from build123d import *

# Parameters (mm, degrees)
SKETCH1_W                        = 55.245
SKETCH1_H                        = 36.15436
BOSS_EXTRUDE1_DEPTH              = 3.175
SKETCH7_W                        = 3.302
SKETCH7_H                        = 19.177
CUT_EXTRUDE1_DEPTH               = 3.175
FILLET1_R                        = 6.35
F_10_0_1935_DIAMETER_HOLE2_D     = 4.9149
F_10_0_1935_DIAMETER_HOLE2_DEPTH = 9.699415072
F_10_0_1935_DIAMETER_HOLE2_TIP   = 1.476584928


with BuildPart() as part:
    # Sketch1 → Boss-Extrude1 (new body)
    with BuildSketch(Plane(origin=(0, 0, 0), x_dir=(0, 0, -1), z_dir=(1, 0, 0))):
        with Locations((27.6225, 18.07718)):
            Rectangle(SKETCH1_W, SKETCH1_H)
    extrude(amount=BOSS_EXTRUDE1_DEPTH)

    # Sketch7 → Cut-Extrude1 (cut)
    with BuildSketch(Plane.ZY):
        with Locations((-43.469153092, 20.34286)):
            Rectangle(SKETCH7_W, SKETCH7_H)
        with Locations((-17.942153092, 20.34286)):
            Rectangle(SKETCH7_W, SKETCH7_H)
    extrude(amount=-CUT_EXTRUDE1_DEPTH, mode=Mode.SUBTRACT)

    # Fillet1
    fillet1_edges = [part.edges().sort_by_distance(p)[0] for p in [
        (1.5875, 0, 0),
        (1.5875, 36.15436, 0),
        (1.5875, 36.15436, -55.245),
        (1.5875, 0, -55.245),
    ]]
    fillet(fillet1_edges, radius=FILLET1_R)

    # #10 (0.1935) Diameter Hole2
    with Locations(Plane.ZY):
        with Locations((-30.642153092, 9.525), (-30.642153092, 26.67), (-6.829653092, 9.525)):
            Hole(F_10_0_1935_DIAMETER_HOLE2_D / 2, depth=F_10_0_1935_DIAMETER_HOLE2_DEPTH)
            with Locations((0, 0, -(F_10_0_1935_DIAMETER_HOLE2_DEPTH + F_10_0_1935_DIAMETER_HOLE2_TIP / 2))):  # 118° drill point
                Cone(0, F_10_0_1935_DIAMETER_HOLE2_D / 2, F_10_0_1935_DIAMETER_HOLE2_TIP, mode=Mode.SUBTRACT)


solid = part.part
Build history of the part. All positions in model axes, mm. A direction names the side the tool comes from. Give positions to 0.01 mm unless a question says otherwise; leave off trailing zeros. Loops run counter-clockwise (first coordinate to the right, second up) from the corner with the lowest first, then second, coordinate; pieces in that order, holes last. Notation, with made-up numbers: (-10, 65.5) - (40, 65.5) arc R26 cw to (40, 100.5) - close; hole circle Ø7 at (29, 69). An arc over 180 degrees is marked (long way). Write item = value, one per line. Start each with the question number.
1) Tool access for faces 4 (the flat face through (2, 18, -55.245)), 5 (the flat face through (2, 10.754, -18)): list every direction of +Z, -Z, +X, -X, +Y, -Y with a clear straight run to the whole face (end or side of a thin tool).
2) Probe probe 1 along Y at (x, z) = (0.5, -30.5); probe 2 along Y at (x, z) = (2.45, -45); probe 3 along Z at (x, y) = (1.8, 19) (3 decimals). List the from-to ranges inside material, lowest first. Write a range as from..to.
3) Band-saw the part on C-C on y = 26.67. Give the cut face in (x, z) (3 decimals), plus the area to 3 significant figures.
4) Band-saw the part on D-D on x = 1.1. Give the cut face in (y, z) (3 decimals).
5) Pull direction Z, two halves, no side cores. Call faces 1 (the flat face through (2, 36.154, -27)), 2 (the cylindrical face through (1.61, 34.245, -1.811)), 3 (the flat face through (2, 29.931, -18)): +Z half, -Z half, draft (parallel to the pull), parting line (faces both ways), or undercut.
6) Band-saw the part on B-B on y = 18. Give the cut face in (x, z) (3 decimals), plus the area to 3 significant figures.
7) Band-saw the part on A-A on z = -18. Give the cut face in (x, y) (3 decimals), plus the area to 3 significant figures.
Final values:
q1.face_4 = -Z, +X, -X, +Y, -Y
q1.face_5 = +X, -X
q2.probe_1 = 0..7.07, 11.98..24.22, 29.12..36.15
q2.probe_2 = 0..10.75, 29.93..36.15
q2.probe_3 = -55.245..-45.12, -41.818..-19.593, -16.291..0
q3.outline = (0, -55.245) - (3.175, -55.245) - (3.175, -45.12) - (0, -45.12) - close; (0, -41.818) - (3.175, -41.818) - (3.175, -33.1) - (0, -33.1) - close; (0, -28.185) - (3.175, -28.185) - (3.175, -19.593) - (0, -19.593) - close; (0, -16.291) - (3.175, -16.291) - (3.175, 0) - (0, 0) - close
q3.area = 139 mm²
q4.outline = (0, -48.895) arc R6.35 ccw to (6.35, -55.245) - (29.804, -55.245) arc R6.35 ccw to (36.154, -48.895) - (36.154, -6.35) arc R6.35 ccw to (29.804, 0) - (6.35, 0) arc R6.35 ccw to (0, -6.35) - close; hole circle Ø4.915 at (9.525, -30.642); hole circle Ø4.915 at (9.525, -6.83); hole (10.754, -45.12) - (29.931, -45.12) - (29.931, -41.818) - (10.754, -41.818) - close; hole (10.754, -19.593) - (29.931, -19.593) - (29.931, -16.291) - (10.754, -16.291) - close; hole circle Ø4.915 at (26.67, -30.642)
q5.face_1 = draft
q5.face_2 = +Z half
q5.face_3 = undercut
q6.outline = (0, -55.245) - (3.175, -55.245) - (3.175, -45.12) - (0, -45.12) - close; (0, -41.818) - (3.175, -41.818) - (3.175, -19.593) - (0, -19.593) - close; (0, -16.291) - (3.175, -16.291) - (3.175, 0) - (0, 0) - close
q6.area = 154 mm²
q7.outline = (0, 0) - (3.175, 0) - (3.175, 10.754) - (0, 10.754) - close; (0, 29.931) - (3.175, 29.931) - (3.175, 36.154) - (0, 36.154) - close
q7.area = 53.9 mm²
